from build123d import *

# Parameters (mm, degrees)
SKETCH1_R           = 11
SKETCH1_R_2         = 4.25
BOSS_EXTRUDE1_DEPTH = 9
SKETCH2_R           = 11
CUT_EXTRUDE1_DEPTH  = 8
SKETCH4_R           = 2
CUT_EXTRUDE2_DEPTH  = 1


with BuildPart() as part:
    # Sketch1 → Boss-Extrude1 (new body)
    with BuildSketch(Plane(origin=(0, 0, 0), x_dir=(1, 0, 0), z_dir=(0, 1, 0))):
        with BuildLine():
            Line((30, 0), (30, 20))
            ThreePointArc((30, 20), (15, 35), (0, 20))
            Line((0, 20), (0, 0))
            Line((0, 0), (30, 0))
        make_face()
        with Locations((15, 20)):
            Circle(SKETCH1_R, mode=Mode.SUBTRACT)
        with Locations((15, 20)):
            Circle(SKETCH1_R)
        with Locations((15, 20)):
            Circle(SKETCH1_R_2, mode=Mode.SUBTRACT)
    extrude(amount=BOSS_EXTRUDE1_DEPTH)

    # Sketch2 → Cut-Extrude1 (cut)
    with BuildSketch(Plane(origin=(0, 9, 0), x_dir=(1, 0, 0), z_dir=(0, 1, 0))):
        with Locations((15, 20)):
            Circle(SKETCH2_R)
    extrude(amount=-CUT_EXTRUDE1_DEPTH, mode=Mode.SUBTRACT)

    # Sketch4 → Cut-Extrude2 (cut)
    with BuildSketch(Plane.XY):
        with Locations((7.5, 4.5)):
            Circle(SKETCH4_R)
        with Locations((22.5, 4.5)):
            Circle(SKETCH4_R)
    extrude(amount=-CUT_EXTRUDE2_DEPTH, mode=Mode.SUBTRACT)


solid = part.part
CAD build for the part. Positions are in the model's coordinates, mm. A direction names the side the tool comes from. Round coordinates to 2 decimals unless told otherwise and drop trailing zeros. Order: outer loops, then holes, each group sorted by start corner. A loop starts at its lowest first (then second) coordinate and runs counter-clockwise, first axis right, second up. Notation, with made-up numbers: (68.25, 13) - (121.25, 13) arc R8 ccw to (121.25, 26) - close; hole circle Ø10 at (11.25, 10). An arc over 180 degrees is marked (long way). Return JSON: item names as keys, results as strings.
(1) Cut at B-B (x = 15). Give the cut face in (y, z), then the cut area to 4 significant figures.
Answer key:
{"outline": "(0, -35) - (9, -35) - (9, -31) - (1, -31) - (1, -24.25) - (0, -24.25) - close; (0, -15.75) - (1, -15.75) - (1, -9) - (9, -9) - (9, 0) - (0, 0) - close", "area": "130.5 mm^2"}
(2) Cut at D-D (z = -12.5). Give the cut face in (x, y).
Answer key:
{"outline": "(0, 0) - (30, 0) - (30, 9) - (23.05, 9) - (23.05, 1) - (6.95, 1) - (6.95, 9) - (0, 9) - close"}
(3) Tool access for faces 1 (the face through (14.08, 0.49, -15.85)), 2 (the face through (5.502, 4.588, -0.493)), 3 (the face through (20, 1, -20)): list every direction of +Z, -Z, +X, -X, +Y, -Y with a clear straight run to the whole face (end or side of a thin tool).
Answer key:
{"face 1": "+Y, -Y", "face 2": "+Z", "face 3": "+Y"}
(4) Wall check: probe 1 along Z at (x, y) = (15, 0.55); probe 2 along X at (y, z) = (0.7, -20); probe 3 along Z at (x, y) = (15, 6.25). Give the ranges that are in metal, low to high. Write a range as from..to.
Answer key:
{"probe 1": "z = -35..-24.25, -15.75..0", "probe 2": "x = 0..10.75, 19.25..30", "probe 3": "z = -35..-31, -9..0"}
(5) Pin check, flat tips, straight feed: pin 1 Ø5 at (x, z) = (15, -20) entering from -Y; pin 2 Ø4.5 at (x, y) = (7, 4) entering from +Z; pin 3 Ø1.2 at (x, y) = (23, 5) entering from +Z; pin 4 Ø1 at (y, z) = (3.5, -29.5) entering from +X. Stop position of each tip, or through.
Answer key:
{"pin 1": "passes through", "pin 2": "stops at z = 0", "pin 3": "stops at z = -1", "pin 4": "stops at x = 27"}
(6) Cut at A-A (y = 4.5). Give the cut face in (x, z).
Answer key:
{"outline": "(0, -20) arc R15 ccw to (30, -20) - (30, 0) - (24.5, 0) - (24.5, -1) - (20.5, -1) - (20.5, 0) - (9.5, 0) - (9.5, -1) - (5.5, -1) - (5.5, 0) - (0, 0) - close; hole circle Ø22 at (15, -20)"}
(7) Pull direction Y, two halves, no side cores. Call faces 4 (the face through (0, 4, -10)), 5 (the face through (22, 5, -1)), 6 (the face through (15, 0, -14)), 7 (the face through (7, 5, -1)): +Y half, -Y half, draft (parallel to the pull), parting line (faces both ways), or undercut.
Answer key:
{"face 4": "draft", "face 5": "undercut", "face 6": "-Y half", "face 7": "undercut"}
(8) Cut at C-C (z = -21). Give the cut face in (x, y), then the cut area to 3 significant figures.
Answer key:
{"outline": "(0.03, 0) - (10.87, 0) - (10.87, 1) - (4.05, 1) - (4.05, 9) - (0.03, 9) - close; (19.13, 0) - (29.97, 0) - (29.97, 9) - (25.95, 9) - (25.95, 1) - (19.13, 1) - close", "area": "85.9 mm^2"}
